from build123d import *

# Parameters (mm, degrees)
PAD_DEPTH    = 28
SKETCH002_W  = 44.1
SKETCH002_H  = 3
PAD001_DEPTH = 93.5
PAD002_DEPTH = 5
PAD003_DEPTH = 5
PAD004_DEPTH = 44.1
SKETCH006_W  = 30
SKETCH006_H  = 70
POCKET_DEPTH = 5


with BuildPart() as part:
    # Sketch → Pad (new body)
    with BuildSketch(Plane.XY):
        Polygon((-4.997332, 9), (-2.497332, 9), (-2.497332, 8), (-2.997332, 8), (-2.997332, 4), (37.102668, 4), (37.102668, 8), (36.602668, 8), (36.602668, 9), (39.102668, 9), (39.102668, 0), (-4.997332, 0), (-4.997332, 4), align=None)
    extrude(amount=PAD_DEPTH)

    # Sketch002 (on Face11 of Pad) → Pad001 (join)
    with BuildSketch(Plane.XZ):
        with Locations((17.052668, 1.5)):
            Rectangle(SKETCH002_W, SKETCH002_H)
    extrude(amount=PAD001_DEPTH)

    # Sketch003 (on Face18 of Pad001) → Pad002 (join, symmetric)
    with BuildSketch(Plane.YZ.offset(9.102668)):
        Polygon((-93.5, 2.9), (-93.5, 13.24805), (-90.5, 13.24805), (-89.114181, 12.674025), (-90.5, 12.1), (-90.5, 2.9), align=None)
    extrude(amount=PAD002_DEPTH, both=True)

    # Sketch004 (on Face18 of Pad001) → Pad003 (join, symmetric)
    with BuildSketch(Plane.YZ.offset(27.252668)):
        Polygon((-93.5, 2.9), (-93.5, 13.24805), (-90.5, 13.24805), (-89.114181, 12.674025), (-90.5, 12.1), (-90.5, 2.9), align=None)
    extrude(amount=PAD003_DEPTH, both=True)

    # Sketch005 (on Face14 of Pad003) → Pad004 (join)
    with BuildSketch(Plane.YZ.offset(39.102668)):
        Polygon((0.1, 28), (-2.9, 25.5), (0.1, 25.5), align=None)
    extrude(amount=-PAD004_DEPTH)

    # Sketch006 (on Face26 of Pad004) → Pocket (cut)
    with BuildSketch(Plane.XY.offset(3)):
        with Locations((17.052668, -46.75)):
            Rectangle(SKETCH006_W, SKETCH006_H)
    extrude(amount=-POCKET_DEPTH, mode=Mode.SUBTRACT)


solid = part.part
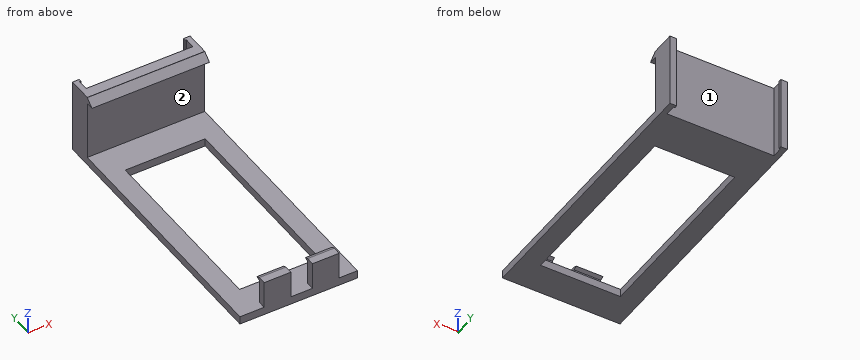
Here's how the part is built. I have some questions about the finished solid (model axes, mm). Face numbers are marked on the shaded views. Round coordinates to 2 decimals unless told otherwise and drop trailing zeros. Loops run counter-clockwise (first coordinate to the right, second up) from the corner with the lowest first, then second, coordinate; pieces in that order, holes last.
1. If we section it at C-C on y = -57.5: Write out the boundary of the cut face in (x, z), plus the area to 3 significant figures.
Answer list:
outline: (-5, 0) - (2.05, 0) - (2.05, 3) - (-5, 3) - close; (32.05, 0) - (39.1, 0) - (39.1, 3) - (32.05, 3) - close
area: 42.3 mm2
2. If we section it at B-B on z = 6: Write out the boundary of the cut face in (x, y).
Answer list:
outline: (-5, 0) - (39.1, 0) - (39.1, 9) - (36.6, 9) - (36.6, 8) - (37.1, 8) - (37.1, 4) - (-3, 4) - (-3, 8) - (-2.5, 8) - (-2.5, 9) - (-5, 9) - close; (4.1, -93.5) - (14.1, -93.5) - (14.1, -90.5) - (4.1, -90.5) - close; (22.25, -93.5) - (32.25, -93.5) - (32.25, -90.5) - (22.25, -90.5) - close
3. For P1, Ø2, axis at y = -91, z = 9, coming from the +X side; P2, Ø1, axis at x = 7, z = 14, coming from the +Y side; P3, Ø6, axis at x = 12.5, z = 22, coming from the -Y side, each with a flat end and sliding along its axis, tell me the tip position at first contact or that it passes through.
Answer list:
P1: stops at x = 32.25
P2: stops at y = 4
P3: stops at y = 0
4. If we section it at D-D on z = 26.75: Write out the boundary of the cut face in (x, y).
Answer list:
outline: (-5, -1.4) - (39.1, -1.4) - (39.1, 9) - (36.6, 9) - (36.6, 8) - (37.1, 8) - (37.1, 4) - (-3, 4) - (-3, 8) - (-2.5, 8) - (-2.5, 9) - (-5, 9) - close
5. If I drill on line 1 along Y through (x, z) = (12.5, 2); line 2 along X through (y, z) = (-50, 1.75); line 3 along Y through (x, z) = (8.5, 10.5), over which ranges is the centre line in solid material (lowest first)?
Answer list:
line 1: y = -93.5 to -81.75, -11.75 to 4
line 2: x = -5 to 2.05, 32.05 to 39.1
line 3: y = -93.5 to -90.5, 0 to 4
6. We'd pull the mould along X, two halves only. Please class the marked faces 1 and 2: +X half, -X half, draft (parallel to the pull), parting line (faces both ways), or undercut.
Answer list:
face 1: undercut
face 2: draft
7. If we section it at A-A on x = 17: Write out the boundary of the cut face in (y, z).
Answer list:
outline: (-93.5, 0) - (-81.75, 0) - (-81.75, 3) - (-93.5, 3) - close; (-11.75, 0) - (4, 0) - (4, 28) - (0, 28) - (0, 27.92) - (-2.9, 25.5) - (0, 25.5) - (0, 3) - (-11.75, 3) - close
